from build123d import *

# Parameters (mm, degrees)
BOSS_EXTRUDE1_DEPTH = 6
CUT_EXTRUDE1_DEPTH  = 51.439717383


with BuildPart() as part:
    # Sketch1 → Boss-Extrude1 (new body)
    # profile 1 of 2: a face of its own
    with BuildSketch(Plane.XY):
        Polygon((31.223066959, -14), (31.223066959, 0), (-34.823066959, 0), (-34.823066959, -4.01574156), (-36.823066959, -3.7), (-41.523066959, -3.7), (-41.523066959, -14), (6.974355653, -28), align=None)
        Polygon((2.700425446, -7.850425446), (2.408714576, -8.979109263), (0.584447895, -7.127556852), (2.009048725, -5.723949904), (3.819278422, -7.561255379), align=None, mode=Mode.SUBTRACT)
    # profile 2 of 2: a face of its own
    with BuildSketch(Plane.XY):
        Polygon((31.223066959, 0), (31.223066959, 14), (6.974355653, 28), (-41.523066959, 14), (-41.523066959, 3.7), (-36.823066959, 3.7), (-34.823066959, 4.01574156), (-34.823066959, 0), align=None)
        Polygon((2.408714576, 8.979109263), (2.700425446, 7.850425446), (3.819278422, 7.561255379), (2.009048725, 5.723949904), (0.584447895, 7.127556852), align=None, mode=Mode.SUBTRACT)
    extrude(amount=BOSS_EXTRUDE1_DEPTH)

    # Sketch2 → Cut-Extrude1 (cut, through all)
    with BuildSketch(Plane.XY.offset(6)):
        Polygon((-41.623066959, -3.427539205), (-41.623066959, -3.8), (-40.023066959, -3.8), (-40.023066959, -6.8), (-38.323066959, -6.8), (-38.323066959, 6.8), (-40.023066959, 6.8), (-40.023066959, 3.8), (-41.623066959, 3.8), (-41.623066959, 3.427539205), align=None)
    extrude(amount=-CUT_EXTRUDE1_DEPTH, mode=Mode.SUBTRACT)


solid = part.part
Could you check a few things on this model? Use its own coordinates, in mm. A direction names the side the tool comes from. Coordinates: 2 decimals unless noted, no trailing zeros. Write each loop counter-clockwise with the first axis right and the second up, starting at its lowest first coordinate (ties: lowest second). Pieces come first, ordered by that corner, then holes. Notation, with made-up numbers: (-23.75, 26.25) - (19.25, 26.25) arc R26 ccw to (19.25, 47.25) - close; hole circle Ø2 at (9.5, -40). An arc over 180 degrees is marked (long way). Write item = value, one per line.
1) Suppose I cut it at B-B on x = -2.5. Please give me the cut outline in (y, z), plus the area to 3 significant figures.
Result set:
outline = (-25.26, 0) - (25.26, 0) - (25.26, 6) - (-25.26, 6) - close
area = 303 mm2
2) For faces 1 (the flat face through (1.287, -6.436, 2.958)), 2 (the flat face through (-38, -3.7, 3)), 3 (the flat face through (-41.523, 9, 3)), which set-ups out of +Z, -Z, +X, -X, +Y, -Y let a thin tool reach every point of the face, with its end or its side?
Result set:
face_1 = +Z, -Z
face_2 = +Z, -Z, -X
face_3 = +Z, -Z, -X, +Y, -Y
3) We'd pull the mould along X, two halves only. Please class faces 4 (the flat face through (-6, 0, 0)), 5 (the flat face through (-38.323, -5, 3)), 6 (the flat face through (19.27, 20.9, 2.96)): +X half, -X half, draft (parallel to the pull), parting line (faces both ways), or undercut.
Result set:
face_4 = draft
face_5 = undercut
face_6 = +X half
4) Suppose I cut it at A-A on z = 1.2. State how many separate pieces and enclosed holes the cut face has, plus the area to 3 significant figures.
Result set:
separate_pieces = 1
enclosed_holes = 2
area = 2,990 mm2
5) Suppose I cut it at C-C on y = -23. Please give me the cut outline in (x, z), plus the area to 3 significant figures.
Result set:
outline = (-10.35, 0) - (15.63, 0) - (15.63, 6) - (-10.35, 6) - close
area = 156 mm2
6) Will these pins go through, and if not, where does the flat tip stop? pin 1 Ø0.8 at (x, z) = (-40.5, 4) entering from +Y; pin 2 Ø1.5 at (x, z) = (18.5, 1) entering from -Y; pin 3 Ø3 at (x, z) = (22.5, 3.5) entering from -Y.
Result set:
pin_1 = 14.41
pin_2 = -21.78
pin_3 = -19.9
7) Please list where these lines run through material, in increasing order: line 1 (Y direction, x = 7, z = 4.1); line 2 (X direction, y = 8.5, z = 4.85); line 3 (X direction, y = -8, z = 3.75). Write a range as [from, to].
Result set:
line_1 = [-27.99, 27.99]
line_2 = [-41.52, 1.94], [2.53, 31.22]
line_3 = [-41.52, 1.44], [2.66, 31.22]
